Check sheet for the modelled part. Datum: model origin and axes. Units: mm. A direction names the side the tool comes from. Coordinates: 2 decimals unless noted, no trailing zeros. Write each loop counter-clockwise with the first axis right and the second up, starting at its lowest first coordinate (ties: lowest second). Pieces come first, ordered by that corner, then holes. Notation, with made-up numbers: (25, 88) - (31, 88) arc R8 cw to (31, 100) - close; hole circle Ø7 at (74.5, 74). An arc over 180 degrees is marked (long way). Write each question's results on one line, items separated by ' | '.
Autodesk Inventor part; units mm, degrees
ref_plane "YZ Plane" through (0, 0, 0) normal (1, 0, 0) x (0, 1, 0)
ref_plane "XZ Plane" through (0, 0, 0) normal (0, 1, 0) x (-1, 0, 0)
ref_plane "XY Plane" through (0, 0, 0) normal (0, 0, 1) x (1, 0, 0)
sketch "Block1" plane through (0, 0, 0) normal (0, 0, 1) x (1, 0, 0)
  circle A0 centre (74.029, 24.2723) radius 1
  line L0 (49.279, 30.4723) -> (71.779, 30.4723)
  line L1 (71.779, 30.4723) -> (71.779, 18.0723)
  line L2 (71.779, 18.0723) -> (49.279, 18.0723)
  line L3 (49.279, 18.0723) -> (49.279, 30.4723)
  line L4 (49.279, 30.4723) -> (44.779, 30.4723)
  line L5 (44.779, 30.4723) -> (44.779, 18.0723)
  line L6 (44.779, 18.0723) -> (49.279, 18.0723)
  line L7 (49.279, 18.0723) -> (49.279, 30.4723)
  line L8 (71.779, 30.4723) -> (76.279, 30.4723)
  line L9 (76.279, 30.4723) -> (76.279, 18.0723)
  line L10 (76.279, 18.0723) -> (71.779, 18.0723)
  line L11 (71.779, 18.0723) -> (71.779, 30.4723)
  line L12 (44.779, 24.2723) -> (76.279, 24.2723) construction
  line L13 (47.029, 30.4723) -> (47.029, 18.0723) construction
  circle A1 centre (47.029, 24.2723) radius 1
  line L14 (74.029, 30.4723) -> (74.029, 18.0723) construction
  point P0 (60.979, 24.0984)
  dimension "d7" = 22.5
  dimension "d8" = 12.4
  dimension "d9" = 4.5
  dimension "d10" = 4.5
  dimension "d11" = 2
  dimension "d12" = 2
sketch "Sketch1" plane through (0, 0, 0) normal (0, 0, 1) x (1, 0, 0)
  line L0 (-92.7646, -8.503) -> (-89.7646, -8.503)
  line L1 (-89.7646, -8.503) -> (-89.7646, -11.753)
  line L2 (-89.7646, -11.753) -> (-92.7646, -11.753)
  line L3 (-92.7646, -11.753) -> (-92.7646, -8.503)
  line L4 (-92.7646, -21.6527) -> (-89.7646, -21.6527)
  line L5 (-89.7646, -21.6527) -> (-89.7646, -21.7527)
  line L6 (-89.7646, -21.7527) -> (-92.7646, -21.7527)
  line L7 (-92.7646, -21.7527) -> (-92.7646, -21.6527)
  line L8 (-66.3097, 47.8088) -> (23.6903, 47.8088)
  line L9 (23.6903, 47.8088) -> (23.6903, 20.8088)
  line L10 (23.6903, 20.8088) -> (-66.3097, 20.8088)
  line L11 (-66.3097, 20.8088) -> (-66.3097, 47.8088)
  line L12 (-66.3097, 34.3088) -> (23.6903, 34.3088) construction
  circle A0 centre (-60.3097, 41.8088) radius 1
  circle A1 centre (-60.3097, 26.8088) radius 1
  line L13 (-31.3097, 41.3088) -> (-28.0597, 41.3088)
  line L14 (-28.0597, 41.3088) -> (-28.0597, 27.3088)
  line L15 (-28.0597, 27.3088) -> (-31.3097, 27.3088)
  line L16 (-31.3097, 27.3088) -> (-31.3097, 41.3088)
  line L17 (-31.3097, 34.3088) -> (-28.0597, 34.3088) construction
  line L18 (-53.3097, 47.8088) -> (-53.3097, 20.8088) construction
  line L19 (-21.3097, 47.8088) -> (-21.3097, 20.8088) construction
  line L20 (10.6903, 47.8088) -> (10.6903, 20.8088) construction
  arc A2 (-53.3097, 47.8088) -> (-53.3097, 20.8088) centre (-52.8001, 34.3088) ccw
  arc A3 (10.6903, 20.8088) -> (10.6903, 47.8088) centre (10.1806, 34.3088) ccw
  circle A4 centre (-10.5597, 34.3088) radius 1
  line L21 (14.1903, 28.1088) -> (-8.3097, 28.1088)
  line L22 (-8.3097, 28.1088) -> (-8.3097, 40.5088)
  line L23 (-8.3097, 40.5088) -> (14.1903, 40.5088)
  line L24 (14.1903, 40.5088) -> (14.1903, 28.1088)
  line L25 (14.1903, 28.1088) -> (18.6903, 28.1088)
  line L26 (18.6903, 28.1088) -> (18.6903, 40.5088)
  line L27 (18.6903, 40.5088) -> (14.1903, 40.5088)
  line L28 (14.1903, 40.5088) -> (14.1903, 28.1088)
  line L29 (-8.3097, 28.1088) -> (-12.8097, 28.1088)
  line L30 (-12.8097, 28.1088) -> (-12.8097, 40.5088)
  line L31 (-12.8097, 40.5088) -> (-8.3097, 40.5088)
  line L32 (-8.3097, 40.5088) -> (-8.3097, 28.1088)
  line L33 (18.6903, 34.3088) -> (-12.8097, 34.3088) construction
  line L34 (16.4403, 28.1088) -> (16.4403, 40.5088) construction
  circle A5 centre (16.4403, 34.3088) radius 1
  line L35 (-10.5597, 28.1088) -> (-10.5597, 40.5088) construction
  point P0 (0, 0)
  dimension "d0" = 3
  dimension "mat" = 3.25
  dimension "d2" = 3
  dimension "d3" = 0.1
  dimension "d23" = 90
  dimension "d24" = 27
  dimension "d25" = 5
  dimension "d26" = 2
  dimension "d27" = 5
  dimension "d28" = 5
  dimension "d29" = 3.25
  dimension "d30" = 14
  dimension "d31" = 35
  dimension "d36" = 13
  dimension "d38" = 13
extrude "Extrusion4" add sketch "Sketch1" along normal blind 3.25 contours L8 A3 L10 A2 | L24 L27 L26 L25 | L29 L30 L31 L22
equation "\"d29\" = mat"
equation "\"d40\" = mat"
properties part number "arm-servo"
1. Sectioned sample at B-B (y = 31.5). Give the number of separate pieces and of enclosed holes in the cut face, then the cut area to 3 significant figures.
Values follow:
separate pieces: 3 | enclosed holes: 0 | area: 207 mm^2
2. Sectioned sample at D-D (y = 43.75). Record the cut outline in (x, z).
Values follow:
outline: (-62.46, 0) - (19.84, 0) - (19.84, 3.25) - (-62.46, 3.25) - close
3. Access from +Z, -Z, +X, -X, +Y, -Y to the whole of each face (thin tool, end or side, straight path). Record for faces 5 (the flat face through (-28.06, 34, 2)), 6 (the cylindrical face through (-66.307, 34.019, 1.602)).
Values follow:
face 5: +Z, -Z | face 6: +Z, -Z, -X
4. Sectioned sample at A-A (x = 7). Record the cut outline in (y, z).
Values follow:
outline: (20.81, 0) - (28.11, 0) - (28.11, 3.25) - (20.81, 3.25) - close; (40.51, 0) - (47.81, 0) - (47.81, 3.25) - (40.51, 3.25) - close
5. Material ranges on L1, parallel to X at y = 37.25, z = 2.1; L2, parallel to X at y = 40.25, z = 0.9; L3, parallel to Y at x = 7, z = 1.85, recorded low to high. Write a range as [from, to].
Values follow:
L1: x = [-65.99, -31.31], [-28.06, -8.31], [14.19, 23.37] | L2: x = [-64.93, -31.31], [-28.06, -8.31], [14.19, 22.31] | L3: y = [20.81, 28.11], [40.51, 47.81]
6. Sectioned sample at C-C (z = 2.55). Record the cut outline in (x, y).
Values follow:
outline: (-53.31, 20.81) - (10.69, 20.81) arc R13.51 ccw to (10.69, 47.81) - (-53.31, 47.81) arc R13.51 ccw to start; hole circle Ø2 at (-60.31, 26.81); hole circle Ø2 at (-60.31, 41.81); hole (-31.31, 27.31) - (-28.06, 27.31) - (-28.06, 41.31) - (-31.31, 41.31) - close; hole circle Ø2 at (-10.56, 34.31); hole (-8.31, 28.11) - (14.19, 28.11) - (14.19, 40.51) - (-8.31, 40.51) - close; hole circle Ø2 at (16.44, 34.31)
7. Go/stop test with flat-tipped pins: pin 1 (1 mm diameter, centred on y = 35.5, z = 1, fed in from -X); pin 2 (1 mm diameter, centred on y = 32, z = 1, fed in from +X). Record where each tip stops, or that it passes through.
Values follow:
pin 1: stops at x = -66.29 | pin 2: stops at x = 23.57
8. Draft check along Y on faces 1 (the flat face through (-22, 47.809, 2)), 2 (the cylindrical face through (23.687, 34.599, 1.602)), 3 (the flat face through (-22, 34, 0)), 4 (the cylindrical face through (-10.776, 35.285, 1.602)). Enter one of: pulls with the +Y half, pulls with the -Y half, needs draft (parallel to the pull), parting line crosses it, or undercut.
Values follow:
face 1: pulls with the +Y half | face 2: parting line crosses it | face 3: needs draft | face 4: undercut
